from build123d import *

# Parameters (mm, degrees)
SKETCH1_R           = 2.5
BOSS_EXTRUDE1_DEPTH = 26
SKETCH2_R           = 7.5
BOSS_EXTRUDE2_DEPTH = 2
FILLET1_R           = 1


with BuildPart() as part:
    # Sketch1 → Boss-Extrude1 (new body)
    with BuildSketch(Plane(origin=(0, 0, 0), x_dir=(1, 0, 0), z_dir=(0, 1, 0))):
        with Locations(Location((0, 0, 0), (0, 0, 90))):
            Circle(SKETCH1_R)
    extrude(amount=BOSS_EXTRUDE1_DEPTH)

    # Sketch2 → Boss-Extrude2 (add)
    with BuildSketch(Plane(origin=(0, 26, 0), x_dir=(1, 0, 0), z_dir=(0, 1, 0))):
        with Locations(Location((0, 0, 0), (0, 0, 270))):
            Circle(SKETCH2_R)
    extrude(amount=BOSS_EXTRUDE2_DEPTH)

    # Fillet1
    fillet1_edges = [part.edges().sort_by_distance(p)[0] for p in [
        (0, 26, -7.5),
        (0, 28, -7.5),
    ]]
    fillet(fillet1_edges, radius=FILLET1_R - 0.0001)  # a hair under: the kernel refuses the full size

    # Mirror1: part across plane


with BuildPart() as part_1:
    add(part.part)
    add(part.part.mirror(Plane.ZX))


solid = part_1.part
Work out the finished part from the listing and answer in its coordinate system (mm). A direction names the side the tool comes from. Give positions to 0.01 mm unless a question says otherwise; leave off trailing zeros. Loops run counter-clockwise (first coordinate to the right, second up) from the corner with the lowest first, then second, coordinate; pieces in that order, holes last. Notation, with made-up numbers: (64.25, -32) -> (122.25, -32) arc R34 ccw to (122.25, -2) -> close; hole circle Ø7 at (13, 35). An arc over 180 degrees is marked (long way). Use a Markdown table: item, result. Add a question column.
1) The part is cut by section C-C, the plane y = -18.5. Determine the outline of the cut face in (x, z).
2) Consider line 1 along Y through (x, z) = (-3.5, -3); line 2 along X through (y, z) = (13.5, 0); line 3 along Z through (x, y) = (0.25, 2). Determine where each line is inside the solid, lowest interval first.
3) Which of the six approach directions +Z, -Z, +X, -X, +Y, -Y give full straight-line access (tool end or side, diameter ignored) to faces 1 (the flat face through (0, -26, 3)), 2 (the flat face through (0, -28, 0))?
4) Each of these flat-tipped pins is pushed along its axis until it touches: P1, Ø5, axis at y = -17.5, z = -1, coming from the -X side; P2, Ø1, axis at y = 16, z = -0.5, coming from the +X side; P3, Ø2, axis at x = 3, y = 0.5, coming from the -Z side. Where does it stop, or does it pass through?
Reported:
| question | item | result |
|---|---|---|
| 1 | outline | circle Ø5 at (0, 0) |
| 2 | line 1 | y = -28 to -26, 26 to 28 |
| 2 | line 2 | x = -2.5 to 2.5 |
| 2 | line 3 | z = -2.49 to 2.49 |
| 3 | face 1 | none |
| 3 | face 2 | +Z, -Z, +X, -X, -Y |
| 4 | P1 | stops at x = -2.5 |
| 4 | P2 | stops at x = 2.5 |
| 4 | P3 | stops at z = -1.5 |
